```python
from build123d import *

# Parameters (mm, degrees)
BOSS_EXTRUDE1_DEPTH     = 125
CUT_EXTRUDE1_DEPTH      = 10
CUT_EXTRUDE2_START      = -5
CUT_EXTRUDE2_DEPTH      = 5
CUT_EXTRUDE3_START      = -10
CUT_EXTRUDE3_DEPTH      = 10
FILLET1_R               = 10
CUT_EXTRUDE5_DEPTH      = 154.180898585
CUT_EXTRUDE5_DEPTH_BACK = 154.180898585
SKETCH6_W               = 40
SKETCH6_H               = 35
BOSS_EXTRUDE2_DEPTH     = 15
CUT_EXTRUDE6_DEPTH      = 157.90664054
CUT_EXTRUDE6_DEPTH_BACK = 157.90664054
SKETCH8_R               = 5


with BuildPart() as part:
    # Sketch1 → Boss-Extrude1 (new body)
    with BuildSketch(Plane(origin=(0, 0, 0), x_dir=(1, 0, 0), z_dir=(0, 1, 0))):
        with BuildLine():
            Line((0, 0), (-40, 0))
            Line((-40, 0), (-40, -15.82575695))
            ThreePointArc((-40, -15.82575695), (-69.724211568, 35.244309675), (-30, 78.989794856))
            Line((-30, 78.989794856), (-30, 63.989794856))
            Line((-30, 63.989794856), (-25, 63.989794856))
            Line((-25, 63.989794856), (-25, 48.989794856))
            Line((-25, 48.989794856), (-30, 48.989794856))
            Line((-30, 48.989794856), (-30, 15))
            Line((-30, 15), (0, 15))
            Line((0, 15), (0, 0))
        make_face()
    extrude(amount=BOSS_EXTRUDE1_DEPTH)

    # Sketch2 → Cut-Extrude1 (cut)
    with BuildSketch(Plane.XZ):
        with BuildLine():
            Line((-30, -63.989794856), (-40, -63.989794856))
            Line((-40, -63.989794856), (-40, -48.989794856))
            Line((-40, -48.989794856), (-30, -48.989794856))
            Line((-30, -48.989794856), (-30, -15))
            Line((-30, -15), (0, -15))
            Line((0, -15), (0, 0))
            Line((0, 0), (-40, 0))
            Line((-40, 0), (-40, 15.82575695))
            ThreePointArc((-40, 15.82575695), (-69.724211568, -35.244309675), (-30, -78.989794856))
            Line((-30, -78.989794856), (-30, -63.989794856))
        make_face()
    extrude(amount=-CUT_EXTRUDE1_DEPTH, mode=Mode.SUBTRACT)

    # Sketch3 → Cut-Extrude2 (cut)
    with BuildSketch(Plane(origin=(0, 125, 0), x_dir=(1, 0, 0), z_dir=(0, 1, 0)).offset(CUT_EXTRUDE2_START)):
        with BuildLine():
            Line((0, 5), (-63.301270189, 5))
            ThreePointArc((-63.301270189, 5), (-65.594723232, 50.521238105), (-30, 78.989794856))
            Line((-30, 78.989794856), (-30, 63.989794856))
            Line((-30, 63.989794856), (-25, 63.989794856))
            Line((-25, 63.989794856), (-25, 48.989794856))
            Line((-25, 48.989794856), (-30, 48.989794856))
            Line((-30, 48.989794856), (-30, 15))
            Line((-30, 15), (0, 15))
            Line((0, 15), (0, 5))
        make_face()
    extrude(amount=CUT_EXTRUDE2_DEPTH, mode=Mode.SUBTRACT)

    # Sketch4 → Cut-Extrude3 (cut)
    with BuildSketch(Plane(origin=(0, 120, 0), x_dir=(1, 0, 0), z_dir=(0, 1, 0)).offset(CUT_EXTRUDE3_START)):
        with BuildLine():
            Line((-30, 63.989794856), (-40, 63.989794856))
            Line((-40, 63.989794856), (-40, 48.989794856))
            Line((-40, 48.989794856), (-30, 48.989794856))
            Line((-30, 48.989794856), (-30, 15))
            Line((-30, 15), (0, 15))
            Line((0, 15), (0, 5))
            Line((0, 5), (-63.301270189, 5))
            ThreePointArc((-63.301270189, 5), (-65.594723232, 50.521238105), (-30, 78.989794856))
            Line((-30, 78.989794856), (-30, 63.989794856))
        make_face()
    extrude(amount=CUT_EXTRUDE3_DEPTH, mode=Mode.SUBTRACT)

    # Fillet1
    fillet1_edges = [part.edges().sort_by_distance(p)[0] for p in [
        (-30, 60, -15),
    ]]
    fillet(fillet1_edges, radius=FILLET1_R)

    # Sketch6 → Cut-Extrude5 (cut, two sides: drawn at the far end of the back side and taken through both)
    with BuildSketch(Plane(origin=(-30, 0, 0), x_dir=(0, 0, -1), z_dir=(1, 0, 0)).offset(-CUT_EXTRUDE5_DEPTH_BACK)):
        with Locations((58.989794856, 62.5)):
            Rectangle(SKETCH6_W, SKETCH6_H)
    extrude(amount=CUT_EXTRUDE5_DEPTH + CUT_EXTRUDE5_DEPTH_BACK, mode=Mode.SUBTRACT)

    # Sketch7 → Boss-Extrude2 (add)
    with BuildSketch(Plane(origin=(0, 110, 0), x_dir=(1, 0, 0), z_dir=(0, 1, 0))):
        with BuildLine():
            Line((0, 5), (-68.916774738, 19.64871268))
            ThreePointArc((-68.916774738, 19.64871268), (-66.687130436, 12.102741784), (-63.301270189, 5))
            Line((-63.301270189, 5), (0, 5))
        make_face()
    extrude(amount=BOSS_EXTRUDE2_DEPTH)

    # Sketch8 → Cut-Extrude6 (cut, two sides: drawn at the far end of the back side and taken through both)
    with BuildSketch(Plane(origin=(0, 0, -15), x_dir=(-1, 0, 0), z_dir=(0, 0, -1)).offset(-CUT_EXTRUDE6_DEPTH_BACK)):
        with BuildLine():
            Line((15, 20), (15, 100))
            ThreePointArc((15, 100), (10, 95), (5, 100))
            Line((5, 100), (5, 20))
            ThreePointArc((5, 20), (10, 25), (15, 20))
        make_face()
        with Locations((10, 100)):
            Circle(SKETCH8_R)
        with Locations((10, 20)):
            Circle(SKETCH8_R)
    extrude(amount=CUT_EXTRUDE6_DEPTH + CUT_EXTRUDE6_DEPTH_BACK, mode=Mode.SUBTRACT)


solid = part.part
```
Here's how the part is built. I have some questions about the finished solid (model axes, mm). A direction names the side the tool comes from. Round coordinates to 2 decimals unless told otherwise and drop trailing zeros. Loops run counter-clockwise (first coordinate to the right, second up) from the corner with the lowest first, then second, coordinate; pieces in that order, holes last. Notation, with made-up numbers: (45, -10) -> (101, -10) arc R27 ccw to (101, 21) -> close; hole circle Ø9 at (39, 48.25). An arc over 180 degrees is marked (long way). Answer as CSV lines item,"result". Start each with the question number.
1. If we mould it in two halves opening along Y, with no side actions, what happens to faces 1 (the face through (-29, 104, -48.99)), 2 (the face through (-32, 120, -57)), 3 (the face through (-5, 61, -7)), 4 (the face through (-50, 62, -38.99))? For each: pulls with the +Y half, pulls with the -Y half, needs draft (parallel to the pull), parting line crosses it, or undercut.
2. I need wall thicknesses on probe 1 along Y at (x, z) = (-35, -42); probe 2 along Y at (x, z) = (-20.5, -4); probe 3 along X at (y, z) = (72, -29). Which ranges of each line are inside material? Lowest first, please. Write a range as from..to.
3. Imagine slicing it at D-D on y = 103. Write out the boundary of the cut face in (x, z), plus the area to 3 significant figures.
4. I'm going to push flat-ended pins straight in: P1, Ø8, axis at y = 42, z = 11.5, coming from the +X side; P2, Ø2, axis at y = 16, z = -59.5, coming from the +X side; P3, Ø12, axis at y = 20.5, z = -72.5, coming from the +X side. Where does each tip first touch, or does it pass through?
5. Imagine slicing it at A-A on y = 36. Write out the boundary of the cut face in (x, z), plus the area to 3 significant figures.
6. Imagine slicing it at B-B on x = -10. Write out the boundary of the cut face in (y, z).
7. For faces 5 (the face through (-40, 115, -57)), 6 (the face through (-42, 45, -54)), 7 (the face through (-17, 59, -15)), 8 (the face through (-10, 105, -7)), 9 (the face through (-29, 17, -48.99)), which set-ups out of +Z, -Z, +X, -X, +Y, -Y let a thin tool reach every point of the face, with its end or its side?
8. Imagine slicing it at C-C on z = -41. Write out the boundary of the cut face in (x, y) (3 decimals).
Solution:
1,face 1,"needs draft"
1,face 2,"pulls with the +Y half"
1,face 3,"undercut"
1,face 4,"undercut"
2,probe 1,"10..45, 80..110"
2,probe 2,"10..125"
2,probe 3,"-69.99..-30"
3,outline,"(-40, 0) -> (-40, 15.83) arc R50 ccw to (-30, -78.99) -> (-30, -63.99) -> (-25, -63.99) -> (-25, -48.99) -> (-30, -48.99) -> (-30, -25) arc R10 cw to (-20, -15) -> (-14, -15) -> (-14, 0) -> close; (-6, -15) -> (0, -15) -> (0, 0) -> (-6, 0) -> close"
3,area,"3,180 mm²"
4,P1,"x = -40"
4,P2,"x = -25"
4,P3,"x = -30"
5,outline,"(-40, 0) -> (-40, 15.83) arc R50 ccw to (-30, -78.99) -> (-30, -63.99) -> (-25, -63.99) -> (-25, -48.99) -> (-30, -48.99) -> (-30, -25) arc R10 cw to (-20, -15) -> (-15, -15) -> (-15, 0) -> close; (-5, -15) -> (0, -15) -> (0, 0) -> (-5, 0) -> close"
5,area,"3,150 mm²"
6,outline,"(10, -15) -> (15, -15) -> (15, 0) -> (10, 0) -> close; (105, -15) -> (110, -15) -> (110, -7.13) -> (125, -7.13) -> (125, 0) -> (105, 0) -> close"
7,face 5,"-Z, -X, +Y"
7,face 6,"-Z, +X, -X"
7,face 7,"-Z, +X, +Y, -Y"
7,face 8,"+Z, -Z"
7,face 9,"+X, -Y"
8,outline,"(-68.775, 10) -> (-30, 10) -> (-30, 45) -> (-68.775, 45) -> close; (-68.775, 80) -> (-30, 80) -> (-30, 110) -> (-68.775, 110) -> close"
